Can you work these out from the drawing? Everything is in mm from the part's minimum corner. Coordinates: 2 decimals unless noted, no trailing zeros. Write each loop counter-clockwise with the first axis right and the second up, starting at its lowest first coordinate (ties: lowest second). Pieces come first, ordered by that corner, then holes. Notation, with made-up numbers: (14, 82.25) -> (47, 82.25) arc R9 cw to (47, 92.25) -> close; hole circle Ø7 at (35.5, 9.25). An arc over 180 degrees is marked (long way). Answer as CSV lines item,"result". Start each with the question number.
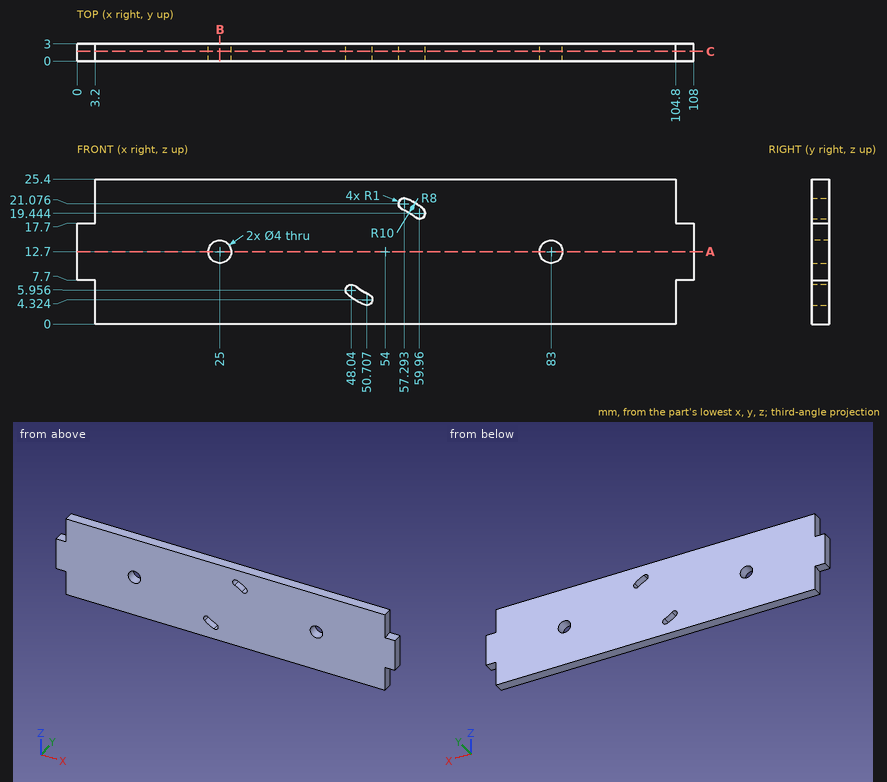
Q1. For pin 1 (3.5 mm diameter, centred on x = 25, z = 12.7, fed in from -Y); pin 2 (0.9 mm diameter, centred on x = 106.5, y = 1, fed in from -Z); pin 3 (1.5 mm diameter, centred on x = 107, y = 1.5, fed in from +Z); pin 4 (0.9 mm diameter, centred on y = 1.5, z = 20.5, fed in from -X), each with a flat end and sliding along its axis, tell me the tip position at first contact or that it passes through.
Q2. Imagine slicing it at B-B (x = 25). Write out the boundary of the cut face in (y, z), then the cut area to 3 significant figures.
Q3. Imagine slicing it at C-C (y = 1.7). Write out the boundary of the cut face in (x, z) (1 decimal).
Q4. I need wall thicknesses on L1, parallel to X at y = 0.9, z = 12.7; L2, parallel to Z at x = 83, y = 1.25; L3, parallel to X at y = 1.5, z = 1.25. Which ranges of each line are inside material? Lowest first, please.
Q5. Imagine slicing it at A-A (z = 12.7). Write out the boundary of the cut face in (x, y).
Entries:
1,pin 1,"through"
1,pin 2,"z = 7.7"
1,pin 3,"z = 17.7"
1,pin 4,"x = 3.2"
2,outline,"(0, 0) -> (3, 0) -> (3, 10.7) -> (0, 10.7) -> close; (0, 14.7) -> (3, 14.7) -> (3, 25.4) -> (0, 25.4) -> close"
2,area,"64.2 mm2"
3,outline,"(0, 7.7) -> (3.2, 7.7) -> (3.2, 0) -> (104.8, 0) -> (104.8, 7.7) -> (108, 7.7) -> (108, 17.7) -> (104.8, 17.7) -> (104.8, 25.4) -> (3.2, 25.4) -> (3.2, 17.7) -> (0, 17.7) -> close; hole circle Ø4 at (25, 12.7); hole (47.4, 5.2) arc R10 ccw to (50.3, 3.4) arc R1 ccw to (51.1, 5.3) arc R8 cw to (48.7, 6.7) arc R1 ccw to start; hole (56.9, 20.1) arc R8 cw to (59.3, 18.7) arc R1 ccw to (60.6, 20.2) arc R10 ccw to (57.7, 22) arc R1 ccw to start; hole circle Ø4 at (83, 12.7)"
4,L1,"0 to 23, 27 to 81, 85 to 108"
4,L2,"0 to 10.7, 14.7 to 25.4"
4,L3,"3.2 to 104.8"
5,outline,"(0, 0) -> (23, 0) -> (23, 3) -> (0, 3) -> close; (27, 0) -> (81, 0) -> (81, 3) -> (27, 3) -> close; (85, 0) -> (108, 0) -> (108, 3) -> (85, 3) -> close"
